from build123d import *

# Parameters (mm, degrees)
CASE_SKETCH_W      = 40.3
CASE_SKETCH_H      = 38.7
CASE_2_DEPTH       = 10.1
TABS_SKETCH_W      = 8.1
TABS_SKETCH_H      = 2.5
TABS_DEPTH         = 10.1
SHAFT_SKETCH_W     = 3
SHAFT_SKETCH_H     = 4
TAB_HOLES_SKETCH_R = 1.6
TAB_HOLES_DEPTH    = 52.7


with BuildPart() as part:
    # Case Sketch → Case 2 (new, symmetric)
    with BuildSketch(Plane.XY):
        with Locations((10.1, 23.35)):
            Rectangle(CASE_SKETCH_W, CASE_SKETCH_H)
    extrude(amount=CASE_2_DEPTH, both=True)

    # Tabs Sketch → Tabs (add, symmetric)
    with BuildSketch(Plane.XY):
        with Locations((-14.1, 13.45)):
            Rectangle(TABS_SKETCH_W, TABS_SKETCH_H)
        with Locations((34.3, 13.45)):
            Rectangle(TABS_SKETCH_W, TABS_SKETCH_H)
    extrude(amount=TABS_DEPTH, both=True)

    # Shaft Sketch → Shaft (revolve)
    with BuildSketch(Plane.XY, mode=Mode.PRIVATE) as shaft_sk:
        with Locations((1.5, 2)):
            Rectangle(SHAFT_SKETCH_W, SHAFT_SKETCH_H)
    revolve(shaft_sk.sketch.rotate(Axis((0, -500, 0), (0, 1, 0)), 90), axis=Axis((0, -500, 0), (0, 1, 0)))

    # Tab Holes Sketch → Tab Holes (cut, symmetric)
    with BuildSketch(Plane(origin=(0, 0, 0), x_dir=(1, 0, 0), z_dir=(0, 1, 0))):
        with Locations(Location((-14.65, -5, 0), (0, 0, 270))):
            Circle(TAB_HOLES_SKETCH_R)
        with Locations(Location((-14.65, 5, 0), (0, 0, 270))):
            Circle(TAB_HOLES_SKETCH_R)
        with Locations(Location((34.85, -5, 0), (0, 0, 270))):
            Circle(TAB_HOLES_SKETCH_R)
        with Locations(Location((34.85, 5, 0), (0, 0, 270))):
            Circle(TAB_HOLES_SKETCH_R)
    extrude(amount=TAB_HOLES_DEPTH, both=True, mode=Mode.SUBTRACT)


solid = part.part
Design review of the part built by this model. Coordinates are the model's own, in mm. A direction names the side the tool comes from. Give positions to 0.01 mm unless a question says otherwise; leave off trailing zeros. Loops run counter-clockwise (first coordinate to the right, second up) from the corner with the lowest first, then second, coordinate; pieces in that order, holes last. Notation, with made-up numbers: M -10,84.5 L 4,84.5 A16 ccw 4,112.5 Z; hole C 33,89.25 d1. An arc over 180 degrees is marked long. One line per question, with ' | ' between items. Start each with the question number.
1. Add section B-B (x = 34.85). Write out the cut boundary in (y, z).
2. Add section D-D (z = -1.5). Write out the cut boundary in (x, y).
3. To check wall thickness, follow L1, parallel to X at y = 14, z = 5; L2, parallel to Z at x = -14.65, y = 13.4; L3, parallel to Z at x = 34, y = 13. State the ranges of each line that lie inside material, in increasing order.
4. Insertion check: P1, Ø3, axis at y = 23.5, z = 6.5, coming from the -X side; P2, Ø9, axis at x = 34.5, z = -4, coming from the -Y side; P3, Ø1, axis at y = 36.5, z = 2.5, coming from the -X side. Each pin has a flat end and moves straight along its axis. Give the tip position at first contact, or say it passes through.
5. The part is to be moulded in two halves that separate along X. For faces 1 (the face through (-13.064, 13.432, 4.792)), 2 (the face through (30.25, 8, 0)), 3 (the face through (-18.15, 13, 0)), say which applies: released by +X, released by -X, zero draft, split by the parting line, or undercut.
6. For faces 4 (the face through (-14, 14.7, 0)), 5 (the face through (-10.05, 8, 0)), 6 (the face through (34, 12.2, 0)), list the 3-axis set-ups (+Z, -Z, +X, -X, +Y, -Y) from which the entire face can be reached by the end or side of a thin tool; tool diameter is ignored.
7. Add section A-A (z = 5). Write out the cut boundary in (x, y), plus the area to 3 significant figures.
8. Add section C-C (y = 39). Write out the cut boundary in (x, z), plus the area to 3 significant figures.
Worked out:
1) outline: M 12.2,-10.1 L 14.7,-10.1 L 14.7,-6.6 L 12.2,-6.6 Z; M 12.2,-3.4 L 14.7,-3.4 L 14.7,3.4 L 12.2,3.4 Z; M 12.2,6.6 L 14.7,6.6 L 14.7,10.1 L 12.2,10.1 Z
2) outline: M -18.15,12.2 L -10.05,12.2 L -10.05,4 L -2.6,4 L -2.6,0 L 2.6,0 L 2.6,4 L 30.25,4 L 30.25,12.2 L 38.35,12.2 L 38.35,14.7 L 30.25,14.7 L 30.25,42.7 L -10.05,42.7 L -10.05,14.7 L -18.15,14.7 Z
3) L1: x = -18.15 to -16.25, -13.05 to 33.25, 36.45 to 38.35 | L2: z = -10.1 to -6.6, -3.4 to 3.4, 6.6 to 10.1 | L3: z = -10.1 to -6.36, -3.64 to 3.64, 6.36 to 10.1
4) P1: stops at x = -10.05 | P2: stops at y = 4 | P3: stops at x = -10.05
5) face 1: undercut | face 2: released by +X | face 3: released by -X
6) face 4: +Z, -Z, -X, +Y | face 5: +Z, -Z, -X, -Y | face 6: +Z, -Z, +X, -Y
7) outline: M -18.15,12.2 L -16.25,12.2 L -16.25,14.7 L -18.15,14.7 Z; M -13.05,12.2 L -10.05,12.2 L -10.05,4 L 30.25,4 L 30.25,12.2 L 33.25,12.2 L 33.25,14.7 L 30.25,14.7 L 30.25,42.7 L -10.05,42.7 L -10.05,14.7 L -13.05,14.7 Z; M 36.45,12.2 L 38.35,12.2 L 38.35,14.7 L 36.45,14.7 Z | area: 1,580 mm²
8) outline: M -10.05,-10.1 L 30.25,-10.1 L 30.25,10.1 L -10.05,10.1 Z | area: 814 mm²
